Read the model definition and answer for the solid it produces. Units are mm, in the model's axes. Face numbers are marked on the shaded views. A direction names the side the tool comes from. Coordinates: 2 decimals unless noted, no trailing zeros. Order: outer loops, then holes, each group sorted by start corner. A loop starts at its lowest first (then second) coordinate and runs counter-clockwise, first axis right, second up. Notation, with made-up numbers: (15.25, 23.5) - (63.25, 23.5) arc R23 ccw to (63.25, 39.5) - close; hole circle Ø11 at (55.25, 60). An arc over 180 degrees is marked (long way). Use one line per item in the form item = value.
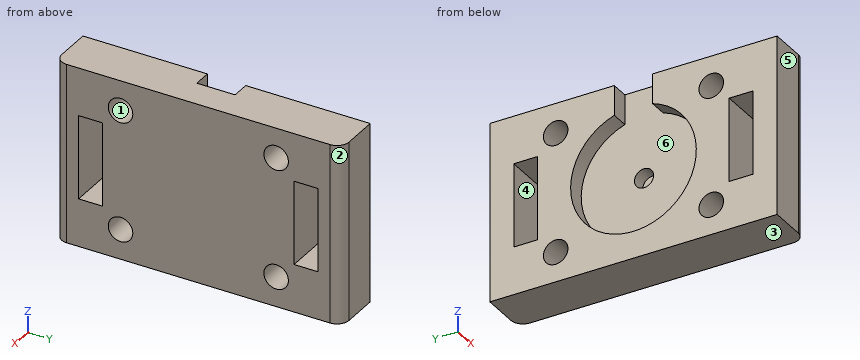
```python
from build123d import *

# Parameters (mm, degrees)
SKETCH1_W                    = 15
SKETCH1_H                    = 24
BOSS_EXTRUDE1_DEPTH          = 4
SKETCH2_R                    = 5.25
CUT_EXTRUDE1_DEPTH           = 1.5
CUT_EXTRUDE2_REACH           = 23.213
CUT_EXTRUDE2_END_RADIUS      = 5.25
SKETCH3_W                    = 1.5
SKETCH3_H                    = 3.2
SKETCH4_R                    = 0.8
CUT_EXTRUDE3_DEPTH           = 1.2
SKETCH5_W                    = 7
SKETCH5_H                    = 2
CUT_EXTRUDE4_DEPTH           = 20.62141687
M2_5X0_45_TAPPED_HOLE1_D     = 2.05
M2_5X0_45_TAPPED_HOLE1_DEPTH = 6.35
M2_5X0_45_TAPPED_HOLE1_TIP   = 0.615882135
FILLET1_R                    = 1


with BuildPart() as part:
    # Sketch1 → Boss-Extrude1 (new body)
    with BuildSketch(Plane(origin=(0, 0, -7.5), x_dir=(0, 0, 1), z_dir=(-1, 0, 0))):
        Rectangle(SKETCH1_W, SKETCH1_H)
    extrude(amount=BOSS_EXTRUDE1_DEPTH)

    # Sketch2 → Cut-Extrude1 (cut)
    with BuildSketch(Plane.ZY.offset(4)):
        with Locations((-7.5, 0)):
            Circle(SKETCH2_R)
    extrude(amount=-CUT_EXTRUDE1_DEPTH, mode=Mode.SUBTRACT)

    # Cut-Extrude2: up to this cylinder (the profile starts outside it)
    cut_extrude2_end = Plane(origin=(-3.25, 0, -7.5), z_dir=(-1, 0, 0)) * Cylinder(CUT_EXTRUDE2_END_RADIUS, 57.926, mode=Mode.PRIVATE)
    # Sketch3 → Cut-Extrude2 (cut, up to the surface)
    with BuildSketch(Plane(origin=(5, 0, 0), x_dir=(1, 0, 0), z_dir=(0, 0, 1)), mode=Mode.PRIVATE) as cut_extrude2_sk1:
        with Locations((-8.25, 0)):
            Rectangle(SKETCH3_W, SKETCH3_H)
    cut_extrude2_tool1 = extrude(cut_extrude2_sk1.sketch, amount=-CUT_EXTRUDE2_REACH, mode=Mode.PRIVATE) - cut_extrude2_end
    add(cut_extrude2_tool1.solids().sort_by_distance((-3.25, 0, 0))[0], mode=Mode.SUBTRACT)

    # Sketch4 → Cut-Extrude3 (cut)
    with BuildSketch(Plane.ZY.offset(2.5)):
        with Locations((-7.5, 0)):
            Circle(SKETCH4_R)
    extrude(amount=-CUT_EXTRUDE3_DEPTH, mode=Mode.SUBTRACT)

    # Sketch5 → Cut-Extrude4 (cut, through all)
    with BuildSketch(Plane.ZY.offset(4)):
        with Locations((-7.5, 9)):
            Rectangle(SKETCH5_W, SKETCH5_H)
        with Locations((-7.5, -9)):
            Rectangle(SKETCH5_W, SKETCH5_H)
    extrude(amount=-CUT_EXTRUDE4_DEPTH, mode=Mode.SUBTRACT)

    # M2.5x0.45 Tapped Hole1
    with Locations(Plane.ZY.offset(4)):
        with Locations((-12.5, -6.5), (-12.5, 6.5), (-2.5, 6.5), (-2.5, -6.5)):
            Hole(M2_5X0_45_TAPPED_HOLE1_D / 2, depth=M2_5X0_45_TAPPED_HOLE1_DEPTH)
            with Locations((0, 0, -(M2_5X0_45_TAPPED_HOLE1_DEPTH + M2_5X0_45_TAPPED_HOLE1_TIP / 2))):  # 118° drill point
                Cone(0, M2_5X0_45_TAPPED_HOLE1_D / 2, M2_5X0_45_TAPPED_HOLE1_TIP, mode=Mode.SUBTRACT)

    # Fillet1
    fillet1_edges = [part.edges().sort_by_distance(p)[0] for p in [
        (0, -12, -7.5),
        (0, 12, -7.5),
    ]]
    fillet(fillet1_edges, radius=FILLET1_R)


solid = part.part
```
(1) Section C-C, the plane z = -7.5 is taken. Write down the section's boundary in (x, y).
Answer list:
outline = (-4, -12) - (-1, -12) arc R1 ccw to (0, -11) - (0, -10) - (-4, -10) - close; (-4, -8) - (0, -8) - (0, 8) - (-4, 8) - (-4, 5.25) - (-2.5, 5.25) - (-2.5, 0.8) - (-1.3, 0.8) - (-1.3, -0.8) - (-2.5, -0.8) - (-2.5, -5.25) - (-4, -5.25) - close; (-4, 10) - (0, 10) - (0, 11) arc R1 ccw to (-1, 12) - (-4, 12) - close
(2) Section B-B, the plane x = -2.9 is taken. Write down the section's boundary in (y, z) (3 decimals).
Answer list:
outline = (-12, -15) - (12, -15) - (12, 0) - (1.6, 0) - (1.6, -2.5) arc R5.25 cw (long way) to (-1.6, -2.5) - (-1.6, 0) - (-12, 0) - close; hole (-10, -11) - (-8, -11) - (-8, -4) - (-10, -4) - close; hole circle Ø2.05 at (-6.5, -12.5); hole circle Ø2.05 at (-6.5, -2.5); hole circle Ø2.05 at (6.5, -12.5); hole circle Ø2.05 at (6.5, -2.5); hole (8, -11) - (10, -11) - (10, -4) - (8, -4) - close
(3) Given pin 1 Ø1.8 at (y, z) = (0, -7.5) entering from -X, flat-ended and moving along its own axis, determine where the tip first touches the part or whether it passes through.
Answer list:
pin_1 = -2.5
(4) Straight lines are drawn through the part: L1, parallel to Y at x = -0.9, z = -12.5 (3 decimals); L2, parallel to Y at x = -1.8, z = -7.5; L3, parallel to Y at x = -1.35, z = -6.5. For each, find the intervals that lie inside material, in ascending order.
Answer list:
L1 = -11.995 to -7.525, -5.475 to 5.475, 7.525 to 11.995
L2 = -12 to -10, -8 to -0.8, 0.8 to 8, 10 to 12
L3 = -12 to -10, -8 to 8, 10 to 12
(5) The mould has two halves that part along Z. Classify the marked faces 1, 2 and 3: +Z half, -Z half, draft (parallel to the pull), parting line (faces both ways), or undercut.
Answer list:
face_1 = undercut
face_2 = draft
face_3 = -Z half
(6) Section A-A, the plane y = 6.5 is taken. Write down the section's boundary in (x, z) (3 decimals), then the cut area to 3 significant figures.
Answer list:
outline = (-4, -15) - (0, -15) - (0, -13.525) - (-4, -13.525) - close; (-4, -11.475) - (0, -11.475) - (0, -3.525) - (-4, -3.525) - close; (-4, -1.475) - (0, -1.475) - (0, 0) - (-4, 0) - close
area = 43.6 mm2
(7) Which of the six approach directions +Z, -Z, +X, -X, +Y, -Y give full straight-line access (tool end or side, diameter ignored) to the marked faces 4, 5 and 6?
Answer list:
face_4 = +X, -X
face_5 = +Z, -Z, +X, -X, -Y
face_6 = -X
(8) Section D-D, the plane y = 0 is taken. Write down the section's boundary in (x, z).
Answer list:
outline = (-4, -15) - (0, -15) - (0, 0) - (-2.5, 0) - (-2.5, -6.7) - (-1.3, -6.7) - (-1.3, -8.3) - (-2.5, -8.3) - (-2.5, -12.75) - (-4, -12.75) - close
